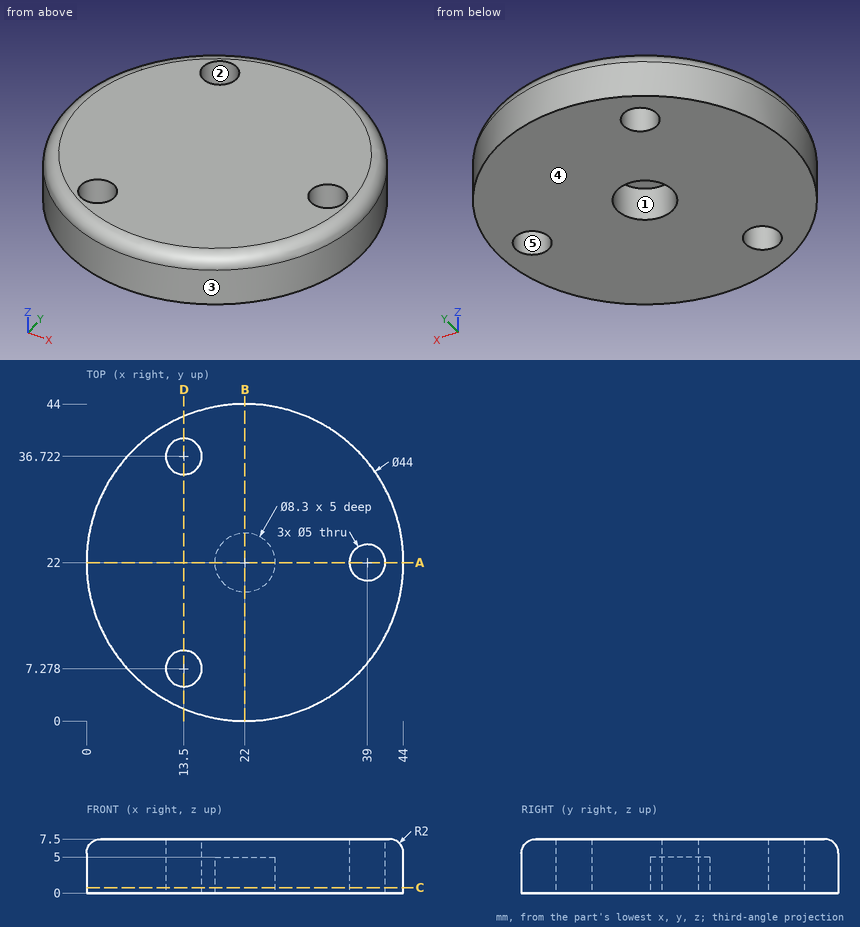
Design review of the part shown in the three views and the two pictorial views. Dimensions are in mm from the part's minimum x, y and z. A direction names the side the tool comes from. Give positions to 0.01 mm unless a question says otherwise; leave off trailing zeros. Loops run counter-clockwise (first coordinate to the right, second up) from the corner with the lowest first, then second, coordinate; pieces in that order, holes last. Notation, with made-up numbers: (37, -19.75) -> (49, -19.75) arc R16 ccw to (49, -2.75) -> close; hole circle Ø8 at (22, -24). An arc over 180 degrees is marked (long way). Answer as a JSON object with one key per item and string values. Group by question number.
Q1. Wall thickness on line 1 along Y through (x, z) = (12, 6) (1 decimal); line 2 along Y through (x, z) = (13.5, 4.5); line 3 along Y through (x, z) = (22, 1.6): over which ranges is each line inside the solid? List them lowest first.
Q2. Take a section at B-B (x = 22). Write out the cut boundary in (y, z).
Q3. Insertion check: pin 1 (1 mm diameter, centred on y = 19, z = 3, fed in from +X); pin 2 (4.5 mm diameter, centred on x = 13.5, y = 7.28, fed in from +Z); pin 3 (2 mm diameter, centred on y = 20, z = 2.5, fed in from +X); pin 4 (1 mm diameter, centred on y = 4.5, z = 2.5, fed in from +X) (1 decimal). Each pin has a flat end and moves straight along its axis. Give the tip position at first contact, or say it passes through.
Q4. Take a section at C-C (z = 0.75). Write out the cut boundary in (x, y), plus the area to 3 significant figures.
Q5. Take a section at A-A (y = 22). Write out the cut boundary in (x, z).
Q6. Take a section at D-D (x = 13.5). State how many separate pieces and enclosed holes the cut face has.
Q7. Draft analysis for pull direction X (two halves, no side actions). For the marked faces 3, 4 and 5, state which applies: pulls with the +X half, pulls with the -X half, needs draft (parallel to the pull), parting line crosses it, or undercut.
Q8. Tool access review of the marked faces 1 and 2: name each direction out of +Z, -Z, +X, -X, +Y, -Y from which nothing blocks a thin tool from reaching the whole face with its end or side.
Answer below:
{
 "1": {"line 1": "y = 2.5 to 5.3, 9.3 to 34.7, 38.7 to 41.5", "line 2": "y = 1.71 to 4.78, 9.78 to 34.22, 39.22 to 42.29", "line 3": "y = 0 to 17.85, 26.15 to 44"},
 "2": {"outline": "(0, 0) -> (17.85, 0) -> (17.85, 5) -> (26.15, 5) -> (26.15, 0) -> (44, 0) -> (44, 5.5) arc R2 ccw to (42, 7.5) -> (2, 7.5) arc R2 ccw to (0, 5.5) -> close"},
 "3": {"pin 1": "stops at x = 43.86", "pin 2": "passes through", "pin 3": "stops at x = 43.98", "pin 4": "stops at x = 36"},
 "4": {"outline": "circle Ø44 at (22, 22); hole circle Ø5 at (13.5, 7.28); hole circle Ø5 at (13.5, 36.72); hole circle Ø8.3 at (22, 22); hole circle Ø5 at (39, 22)", "area": "1,410 mm2"},
 "5": {"outline": "(0, 0) -> (17.85, 0) -> (17.85, 5) -> (26.15, 5) -> (26.15, 0) -> (36.5, 0) -> (36.5, 7.5) -> (2, 7.5) arc R2 ccw to (0, 5.5) -> close; (41.5, 0) -> (44, 0) -> (44, 5.5) arc R2 ccw to (42, 7.5) -> (41.5, 7.5) -> close"},
 "6": {"separate pieces": "3", "enclosed holes": "0"},
 "7": {"face 3": "parting line crosses it", "face 4": "needs draft", "face 5": "undercut"},
 "8": {"face 1": "-Z", "face 2": "+Z, -Z"}
}
